```python
from build123d import *

# Parameters (mm, degrees)
SALIENTE_EXTRUIR1_DEPTH                              = 3.5
AVELLANADO_PARA_TORNILLO_CON_CABEZA_PLAN_D           = 3.4
AVELLANADO_PARA_TORNILLO_CON_CABEZA_PLAN_CSINK_D     = 6.3
AVELLANADO_PARA_TORNILLO_CON_CABEZA_PLAN_CSINK_ANGLE = 90
REDONDEO1_R                                          = 0.3
CROQUIS4_W                                           = 3
CROQUIS4_H                                           = 42
SALIENTE_EXTRUIR2_DEPTH                              = 0.5
CORTAR_EXTRUIR1_DEPTH                                = 2


with BuildPart() as part:
    # Croquis1 → Saliente-Extruir1 (new body)
    with BuildSketch(Plane(origin=(0, 0, 0), x_dir=(1, 0, 0), z_dir=(0, 1, 0))):
        with BuildLine():
            Line((-7.5, 0), (-7.5, -21))
            Line((-7.5, -21), (-21, -21))
            Line((-21, -21), (-21, -12.28))
            Line((-21, -12.28), (-20.5, -12.28))
            Line((-20.5, -12.28), (-20.5, -2.42))
            Line((-20.5, -2.42), (-21, -2.42))
            Line((-21, -2.42), (-21, 21))
            Line((-21, 21), (21, 21))
            Line((21, 21), (21, -2.42))
            Line((21, -2.42), (20.5, -2.42))
            Line((20.5, -2.42), (20.5, -12.28))
            Line((20.5, -12.28), (21, -12.28))
            Line((21, -12.28), (21, -21))
            Line((21, -21), (7.5, -21))
            Line((7.5, -21), (7.5, 0))
            ThreePointArc((7.5, 0), (0, 7.5), (-7.5, 0))
        make_face()
    extrude(amount=-SALIENTE_EXTRUIR1_DEPTH)

    # Avellanado para tornillo con cabeza plana avellanada de M31 (through all)
    with Locations(Plane(origin=(0, 0, 0), x_dir=(1, 0, 0), z_dir=(0, 1, 0))):
        with Locations((-16, 0), (16, 0)):
            CounterSinkHole(AVELLANADO_PARA_TORNILLO_CON_CABEZA_PLAN_D / 2, AVELLANADO_PARA_TORNILLO_CON_CABEZA_PLAN_CSINK_D / 2, counter_sink_angle=AVELLANADO_PARA_TORNILLO_CON_CABEZA_PLAN_CSINK_ANGLE)

    # Redondeo1
    redondeo1_edges = [part.edges().sort_by_distance(p)[0] for p in [
        (14.25, 0, 21),
        (7.5, 0, 10.5),
        (0, 0, -7.5),
        (-7.5, 0, 10.5),
        (-14.25, 0, 21),
        (-21, 0, 16.64),
        (-20.75, 0, 12.28),
        (-20.5, 0, 7.35),
        (-20.75, 0, 2.42),
        (-21, 0, -9.29),
        (0, 0, -21),
        (21, 0, -9.29),
        (20.75, 0, 2.42),
        (20.5, 0, 7.35),
        (20.75, 0, 12.28),
        (21, 0, 16.64),
    ]]
    fillet(redondeo1_edges, radius=REDONDEO1_R)

    # Croquis4 → Saliente-Extruir2 (add)
    with BuildSketch(Plane.XZ.offset(3.5)):
        with Locations((9.5, 0)):
            Rectangle(CROQUIS4_W, CROQUIS4_H)
        with Locations((-9.5, 0)):
            Rectangle(CROQUIS4_W, CROQUIS4_H)
    extrude(amount=SALIENTE_EXTRUIR2_DEPTH)

    # Croquis5 → Cortar-Extruir1 (cut)
    with BuildSketch(Plane.XZ.offset(3.5)):
        with BuildLine():
            Line((-5.5, -9.7), (5.5, -9.7))
            ThreePointArc((5.5, -9.7), (7, -11.2), (5.5, -12.7))
            Line((5.5, -12.7), (-5.5, -12.7))
            ThreePointArc((-5.5, -12.7), (-7, -11.2), (-5.5, -9.7))
        make_face()
    extrude(amount=-CORTAR_EXTRUIR1_DEPTH, mode=Mode.SUBTRACT)


solid = part.part
```
Input: part model. Units: mm. Frame: model coordinates. A direction names the side the tool comes from. Give positions to 0.01 mm unless a question says otherwise; leave off trailing zeros. Order: outer loops, then holes, each group sorted by start corner. A loop starts at its lowest first (then second) coordinate and runs counter-clockwise, first axis right, second up.
1. Line query: probe 1 along Z at (x, y) = (16, -2.25); probe 2 along X at (y, z) = (-2.7, 0.5); probe 3 along X at (y, z) = (-1.45, 3.5). Output: solid intervals per line, ascending.
Computed:
probe 1: z = -21 to -1.7, 1.7 to 21
probe 2: x = -21 to -17.62, -14.38 to -7.5, 7.5 to 14.38, 17.62 to 21
probe 3: x = -20.5 to -7.5, 7.5 to 20.5
2. Draft query along X for faces 1 (the face through (-21, -2, 17)), 2 (the face through (21, -2, -9)), 3 (the face through (0, 0, -9)), 4 (the face through (0.16, -1.88, -7.5)). Return one class per face: released by +X, released by -X, zero draft, split by the parting line, or undercut.
Computed:
face 1: released by -X
face 2: released by +X
face 3: zero draft
face 4: undercut
3. Set-up query: faces 5 (the face through (7.5, -2, 11)), 6 (the face through (0, -3, -12.7)), 7 (the face through (0, -3.5, -9)), 8 (the face through (-20.5, -2, 7)). Return all of +Z, -Z, +X, -X, +Y, -Y with unobstructed straight access to the full face (end or side cutting, diameter ignored); none if empty.
Computed:
face 5: +Z, +Y, -Y
face 6: -Y
face 7: +Z, -Z, -Y
face 8: -X, +Y, -Y
4. Cut plane A-A (z = 8). Return loops of the section in (x, y).
Computed:
outline: (-20.5, -3.5) - (-11, -3.5) - (-11, -4) - (-8, -4) - (-8, -3.5) - (-7.5, -3.5) - (-7.5, -0.3) arc R0.3 ccw to (-7.8, 0) - (-20.2, 0) arc R0.3 ccw to (-20.5, -0.3) - close; (7.5, -3.5) - (8, -3.5) - (8, -4) - (11, -4) - (11, -3.5) - (20.5, -3.5) - (20.5, -0.3) arc R0.3 ccw to (20.2, 0) - (7.8, 0) arc R0.3 ccw to (7.5, -0.3) - close
5. Cut plane C-C (y = -2.05). Return loops of the section in (x, z), and give its area (3 significant figures).
Computed:
outline: (-21, -21) - (21, -21) - (21, 2.42) - (20.5, 2.42) - (20.5, 12.28) - (21, 12.28) - (21, 21) - (7.5, 21) - (7.5, 0) arc R7.5 cw to (-7.5, 0) - (-7.5, 21) - (-21, 21) - (-21, 12.28) - (-20.5, 12.28) - (-20.5, 2.42) - (-21, 2.42) - close; hole circle Ø3.4 at (-16, 0); hole (-5.5, -12.7) - (5.5, -12.7) arc R1.5 ccw to (5.5, -9.7) - (-5.5, -9.7) arc R1.5 ccw to start; hole circle Ø3.4 at (16, 0)
area: 1,290 mm2
6. Pin query (flat end, axial travel): pin 1 Ø1 at (y, z) = (-2.5, 9) entering from +X; pin 2 Ø11 at (x, z) = (-17, -9.5) entering from -Y; pin 3 Ø0.6 at (y, z) = (-4, -5) entering from -X. Return the tip coordinate at first contact, or that it passes through.
Computed:
pin 1: stops at x = 20.5
pin 2: stops at y = -3.5
pin 3: stops at x = -11
7. Cut plane D-D (z = -11.2). Return loops of the section in (x, y), and give its area (3 significant figures).
Computed:
outline: (-21, -3.5) - (-11, -3.5) - (-11, -4) - (-8, -4) - (-8, -3.5) - (-7, -3.5) - (-7, -1.5) - (7, -1.5) - (7, -3.5) - (8, -3.5) - (8, -4) - (11, -4) - (11, -3.5) - (21, -3.5) - (21, -0.3) arc R0.3 ccw to (20.7, 0) - (-20.7, 0) arc R0.3 ccw to (-21, -0.3) - close
area: 122 mm2
8. Cut plane B-B (x = 16). Return loops of the section in (y, z).
Computed:
outline: (-3.5, -21) - (-0.3, -21) arc R0.3 ccw to (0, -20.7) - (0, -3.15) - (-1.45, -1.7) - (-3.5, -1.7) - close; (-3.5, 1.7) - (-1.45, 1.7) - (0, 3.15) - (0, 20.7) arc R0.3 ccw to (-0.3, 21) - (-3.5, 21) - close
